```python
from build123d import *

# Parameters (mm, degrees)
SKETCH1_R          = 3.5
CUT_EXTRUDE1_DEPTH = 10


with BuildPart() as part:
    # Esboço1 → Revolução1 (revolve)
    with BuildSketch(Plane.XY):
        Polygon((-27.999975, 5), (-27.999975, 16), (-28.699975, 16), (-28.699975, 10), (-30.399975, 10), (-30.399975, 16), (-31.099975, 16), (-31.099975, 10), (-32.799975, 10), (-32.799975, 16), (-33.499975, 16), (-33.499975, 10), (-35.199975, 10), (-35.199975, 16), (-35.899975, 16), (-35.899975, 10), (-37.599975, 10), (-37.599975, 16), (-38.299975, 16), (-38.299975, 10), (-39.999975, 10), (-39.999975, 16), (-40.699975, 16), (-40.699975, 10), (-42.399975, 10), (-42.399975, 16), (-43.099975, 16), (-43.099975, 10), (-44.799975, 10), (-44.799975, 16), (-45.499975, 16), (-45.499975, 10), (-47.199975, 10), (-47.199975, 16), (-47.899975, 16), (-47.899975, 10), (-49.599975, 10), (-49.599975, 16), (-50.299975, 16), (-50.299975, 10), (-51.999975, 10), (-51.999975, 16), (-52.699975, 16), (-52.699975, 10), (-54.399975, 10), (-54.399975, 12.9), (-55.099975, 12.9), (-55.099975, 10), (-56.799975, 10), (-56.799975, 12.9), (-59.799975, 12.9), (-59.799975, 10.9), (-65.799975, 10.9), (-65.799975, 12.9), (-69.099975, 12.9), (-69.099975, 5), align=None)
    revolve(axis=Axis((-27.999975, 5, 0), (-1, 0, 0)))

    # Sketch1 → Cut-Extrude1 (cut)
    with BuildSketch(Plane.ZY.offset(69.099975)):
        with Locations((0, 5)):
            Circle(SKETCH1_R)
    extrude(amount=-CUT_EXTRUDE1_DEPTH, mode=Mode.SUBTRACT)


solid = part.part
```
Geometry check sheet. Reference: the model listing, model coordinates, mm. A direction names the side the tool comes from. Round coordinates to 2 decimals unless told otherwise and drop trailing zeros. Use a Markdown table: item, result. Add a question column.
1) Thickness scan on line 1 along Y through (x, z) = (-66.5, 0); line 2 along X through (y, z) = (2.5, -2.25); line 3 along Y through (x, z) = (-51.5, 0). Record the ranges inside material, lowest first.
2) Mould release check, pull along X, two halves, no side actions. Record for faces 3 (the cylindrical face through (-49.95, 2.62, 10.74)), 4 (the flat face through (-44.8, 0, 2)): released by +X, released by -X, zero draft, split by the parting line, or undercut.
3) Gauge pin test, flat ends, axial feed: P1, Ø10, axis at x = -33, z = -6.5, coming from the +Y side; P2, Ø10, axis at x = -41.5, y = 2.5, coming from the -Z side; P3, Ø1, axis at x = -50.5, z = -8.5, coming from the -Y side; P4, Ø1.5, axis at x = -60.5, y = 6, coming from the -Z side. Record the tip position at first contact, or that the pin passes through.
4) Section check A-A (z = -8.75). Count the separate pieces of the cut face and the enclosed holes in it, then the cut area to 3 significant figures.
5) Set-up check for faces 1 (the cylindrical face through (-45.15, 2.62, 10.74)), 2 (the flat face through (-38.3, 7, 5)): record each of +Z, -Z, +X, -X, +Y, -Y from which the full face is reachable in a straight line by a thin tool's end or side.
Established:
| question | item | result |
|---|---|---|
| 1 | line 1 | -2.9 to 1.5, 8.5 to 12.9 |
| 1 | line 2 | -59.1 to -28 |
| 1 | line 3 | 0 to 10 |
| 2 | face 3 | zero draft |
| 2 | face 4 | undercut |
| 3 | P1 | y = 15.9 |
| 3 | P2 | z = -11 |
| 3 | P3 | y = -2.51 |
| 3 | P4 | z = -7.87 |
| 4 | separate pieces | 11 |
| 4 | enclosed holes | 0 |
| 4 | area | 103 mm2 |
| 5 | face 1 | +X, -X |
| 5 | face 2 | none |
